Could you check a few things on this model? Use its own coordinates, in mm. Coordinates: 2 decimals unless noted, no trailing zeros. Order: outer loops, then holes, each group sorted by start corner. A loop starts at its lowest first (then second) coordinate and runs counter-clockwise, first axis right, second up. Notation, with made-up numbers: M 28.5,79.5 L 67.5,79.5 A17 ccw 67.5,95.5 Z; hole C 27.25,53 d1. An arc over 180 degrees is marked long. One line per question, with ' | ' between items. Start each with the question number.
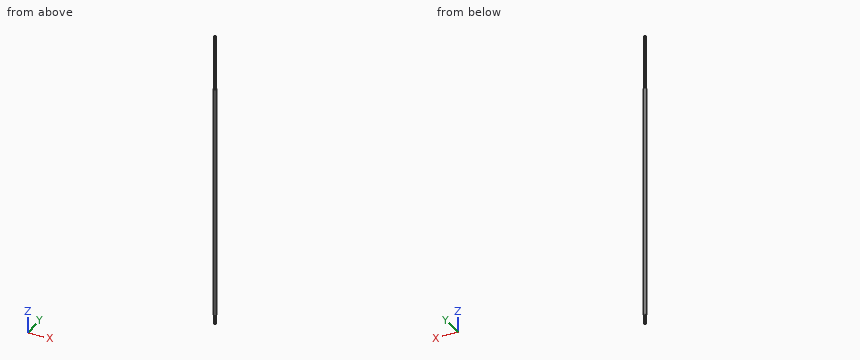
from build123d import *

# Parameters (mm, degrees)
CYLINDER_R      = 4.7625
CYLINDER_DEPTH  = 1219.2
SKETCH_R        = 6
SKETCH_R_2      = 4
POCKET_DEPTH    = 37
SKETCH001_R     = 6
SKETCH001_R_2   = 4
POCKET001_DEPTH = 221


with BuildPart() as part:
    # Cylinder → Cylinder (new body)
    with BuildSketch(Plane.XY):
        Circle(CYLINDER_R)
    extrude(amount=CYLINDER_DEPTH)

    # Sketch → Pocket (cut)
    with BuildSketch(Plane(origin=(0, 0, 0), x_dir=(1, 0, 0), z_dir=(0, 0, -1))):
        Circle(SKETCH_R)
        Circle(SKETCH_R_2, mode=Mode.SUBTRACT)
    extrude(amount=-POCKET_DEPTH, mode=Mode.SUBTRACT)

    # Sketch001 → Pocket001 (cut)
    with BuildSketch(Plane.XY.offset(1219.2)):
        Circle(SKETCH001_R)
        Circle(SKETCH001_R_2, mode=Mode.SUBTRACT)
    extrude(amount=-POCKET001_DEPTH, mode=Mode.SUBTRACT)


solid = part.part
(1) Imagine slicing it at A-A, the plane x = 0. Write out the boundary of the cut face in (y, z), plus the area to 3 significant figures.
(2) For P1, Ø3, axis at y = 0.5, z = 496, coming from the +X side; P2, Ø3, axis at x = -1, z = 1052, coming from the -Y side; P3, Ø2, axis at x = 3.5, z = 1016.5, coming from the +Y side, each with a flat end and sliding along its axis, tell me the tip position at first contact or that it passes through.
(3) If I drill on line 1 along X through (y, z) = (2.5, 462.5); line 2 along Y through (x, z) = (1, 462), over which ranges is the centre line in solid material (lowest first)? Write a range as from..to.
Answers:
1) outline: M -4.76,37 L -4,37 L -4,0 L 4,0 L 4,37 L 4.76,37 L 4.76,998.2 L 4,998.2 L 4,1219.2 L -4,1219.2 L -4,998.2 L -4.76,998.2 Z | area: 11,200 mm²
2) P1: x = 4.76 | P2: y = -4 | P3: y = 3.12
3) line 1: -4.05..4.05 | line 2: -4.66..4.66
